Source: CAD feature listing. Evaluate the final solid. Frame: model axes, mm. Round coordinates to 2 decimals unless told otherwise and drop trailing zeros. Write each loop counter-clockwise with the first axis right and the second up, starting at its lowest first coordinate (ties: lowest second). Pieces come first, ordered by that corner, then holes. Notation, with made-up numbers: M -19,-6 L 33,-6 A18 cw 33,25 Z; hole C 8,57.25 d9. An arc over 180 degrees is marked long. Use a Markdown table: item, result.
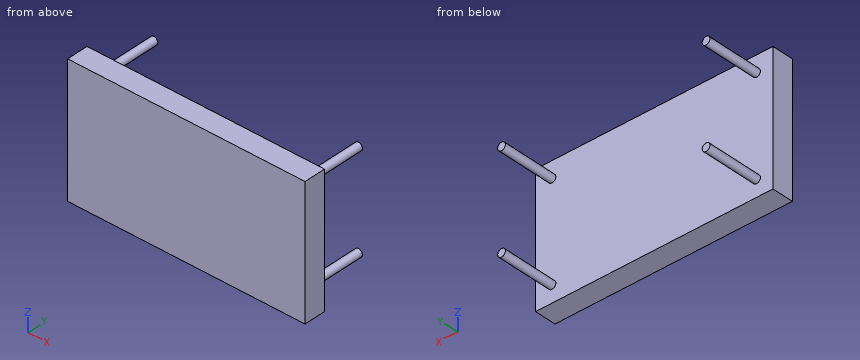
```python
from build123d import *

# Parameters (mm, degrees)
SKETCH1_W           = 55
SKETCH1_H           = 30
BOSS_EXTRUDE1_DEPTH = 5
SKETCH2_R           = 0.9
BOSS_EXTRUDE2_DEPTH = 13


with BuildPart() as part:
    # Sketch1 → Boss-Extrude1 (new body)
    with BuildSketch(Plane(origin=(0, 0, 0), x_dir=(1, 0, 0), z_dir=(0, 1, 0))):
        with Locations((25.5, 13)):
            Rectangle(SKETCH1_W, SKETCH1_H)
    extrude(amount=BOSS_EXTRUDE1_DEPTH)

    # Sketch2 → Boss-Extrude2 (add)
    with BuildSketch(Plane(origin=(0, 5, 0), x_dir=(1, 0, 0), z_dir=(0, 1, 0))):
        with Locations(Location((1.8, 24.2, 0), (0, 0, 90))):
            Circle(SKETCH2_R)
        with Locations(Location((49.2, 24.2, 0), (0, 0, 90))):
            Circle(SKETCH2_R)
        with Locations(Location((49.2, 1.8, 0), (0, 0, 90))):
            Circle(SKETCH2_R)
        with Locations(Location((1.8, 1.8, 0), (0, 0, 90))):
            Circle(SKETCH2_R)
    extrude(amount=BOSS_EXTRUDE2_DEPTH)


solid = part.part
```
Q1. Section A-A on z = -24.2. Return loops of the section in (x, y), plus the area to 3 significant figures.
Results are:
| item | result |
|---|---|
| outline | M -2,0 L 53,0 L 53,5 L 50.1,5 L 50.1,18 L 48.3,18 L 48.3,5 L 2.7,5 L 2.7,18 L 0.9,18 L 0.9,5 L -2,5 Z |
| area | 322 mm^2 |
Q2. Section B-B on x = 1.8. Return loops of the section in (y, z).
Results are:
| item | result |
|---|---|
| outline | M 0,-28 L 5,-28 L 5,-25.1 L 18,-25.1 L 18,-23.3 L 5,-23.3 L 5,-2.7 L 18,-2.7 L 18,-0.9 L 5,-0.9 L 5,2 L 0,2 Z |
Q3. Section C-C on y = 12. Return loops of the section in (x, z).
Results are:
| item | result |
|---|---|
| outline | C 1.8,-24.2 d1.8; C 1.8,-1.8 d1.8; C 49.2,-24.2 d1.8; C 49.2,-1.8 d1.8 |
Q4. Section D-D on z = -8. Return loops of the section in (x, y).
Results are:
| item | result |
|---|---|
| outline | M -2,0 L 53,0 L 53,5 L -2,5 Z |
Q5. Line query: L1, parallel to Y at x = 45.5, z = -11.25; L2, parallel to X at y = 7.75, z = -23.5; L3, parallel to Z at x = 2, y = 7.25. Output: solid intervals per line, ascending.
Results are:
| item | result |
|---|---|
| L1 | 0 to 5 |
| L2 | 1.23 to 2.37, 48.63 to 49.77 |
| L3 | -25.08 to -23.32, -2.68 to -0.92 |
Q6. First-contact query: pin 1 Ø12 at (x, z) = (25, -22.5) entering from -Y. Flat tip, straight axial feed; report the tip coordinate or a pass-through.
Results are:
| item | result |
|---|---|
| pin 1 | y = 0 |
